The model under review builds one solid part; all positions refer to its coordinate system, in mm. Face numbers are marked on the shaded views. Coordinates: 2 decimals unless noted, no trailing zeros. Order: outer loops, then holes, each group sorted by start corner. A loop starts at its lowest first (then second) coordinate and runs counter-clockwise, first axis right, second up. Notation, with made-up numbers: M 81.5,77 L 112.5,77 A31 cw 112.5,114 Z; hole C 1,4.25 d10. An arc over 180 degrees is marked long. Write each question's results on one line, items separated by ' | '.
from build123d import *

# Parameters (mm, degrees)
SKETCH009_W     = 180
SKETCH009_H     = 180
PAD004_DEPTH    = 2
SKETCH010_W     = 178
SKETCH010_H     = 178
PAD005_DEPTH    = 2
SKETCH011_W     = 176
SKETCH011_H     = 176
POCKET003_DEPTH = 2
CHAMFER004_SIZE = 0.5


with BuildPart() as part:
    # Sketch009 → Pad004 (new body)
    with BuildSketch(Plane.XY):
        Rectangle(SKETCH009_W, SKETCH009_H)
    extrude(amount=PAD004_DEPTH)

    # Sketch010 (on DatumPlane) → Pad005 (join)
    with BuildSketch(Plane.XY.offset(2)):
        Rectangle(SKETCH010_W, SKETCH010_H)
    extrude(amount=PAD005_DEPTH)

    # Sketch011 (on DatumPlane) → Pocket003 (cut)
    with BuildSketch(Plane.XY.offset(4)):
        Rectangle(SKETCH011_W, SKETCH011_H)
    extrude(amount=-POCKET003_DEPTH, mode=Mode.SUBTRACT)

    # Chamfer004
    chamfer004_edges = [part.edges().sort_by_distance(p)[0] for p in [
        (0, -90, 2),
        (0, 90, 2),
        (90, 0, 2),
        (-90, 0, 2),
    ]]
    chamfer(chamfer004_edges, length=CHAMFER004_SIZE)


solid = part.part
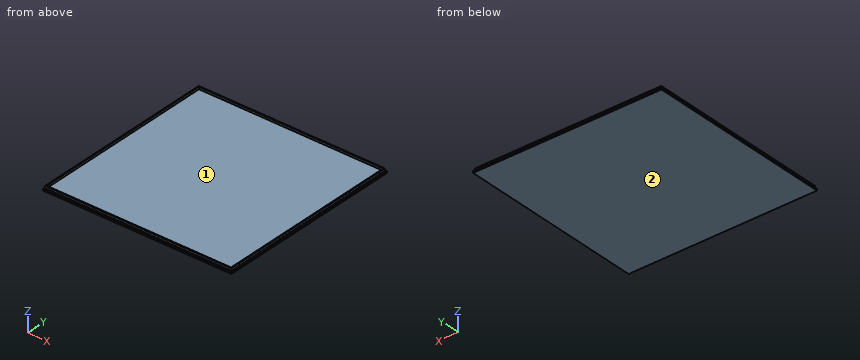
1) The part is to be moulded in two halves that separate along Y. For the marked faces 1 and 2, say which applies: pulls with the +Y half, pulls with the -Y half, needs draft (parallel to the pull), parting line crosses it, or undercut.
Solutions:
face 1: undercut | face 2: needs draft
2) For pin 1 (1.6 mm diameter, centred on y = -21, z = 3, fed in from -X); pin 2 (0.6 mm diameter, centred on y = 12.5, z = 3, fed in from +X); pin 3 (4 mm diameter, centred on x = 2, y = -12.5, fed in from +Z); pin 4 (10 mm diameter, centred on x = -10, y = -30.5, fed in from -Z), all flat-tipped, find the tip position at first contact; note any pin that passes through.
Solutions:
pin 1: x = -89 | pin 2: x = 89 | pin 3: z = 2 | pin 4: z = 0
3) Take a section at A-A on y = 15. State the section outline as (x, z) points.
Solutions:
outline: M -90,0 L 90,0 L 90,1.5 L 89.5,2 L 89,2 L 89,4 L 88,4 L 88,2 L -88,2 L -88,4 L -89,4 L -89,2 L -89.5,2 L -90,1.5 Z
4) To check wall thickness, follow line 1 along Y through (x, z) = (-33, 2.55); line 2 along Z through (x, y) = (75.5, 14). State the ranges of each line that lie inside material, in increasing order.
Solutions:
line 1: -89 to -88, 88 to 89 | line 2: 0 to 2
